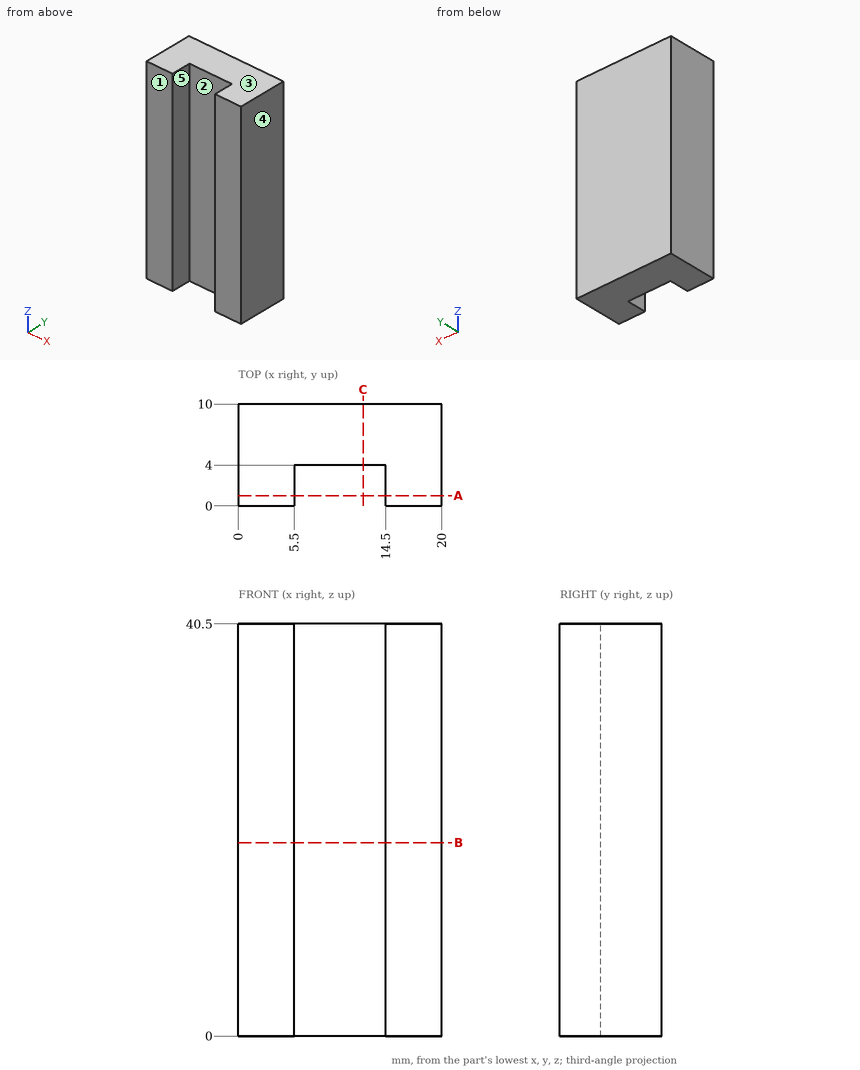
Study the drawing (mm; zero at the part's minimum x, y, z) and answer. A direction names the side the tool comes from. Coordinates: 2 decimals unless noted, no trailing zeros. Write each loop counter-clockwise with the first axis right and the second up, starting at its lowest first coordinate (ties: lowest second). Pieces come first, ordered by that corner, then holes. Notation, with made-up numbers: (49.25, -16.5) -> (76.25, -16.5) arc R20 cw to (76.25, 5.5) -> close; hole circle Ø5 at (20.25, 40). An arc over 180 degrees is marked (long way). Write each question's results on one line, items separated by ' | '. Start each with the question number.
1) A cutting plane is placed at C-C (x = 12.25). Determine the outline of the cut face in (y, z), then the cut area to 3 significant figures.
2) For a pull along X with two mould halves and no side action, classify the marked faces 3, 4 and 5 as +X half, -X half, draft (parallel to the pull), parting line (faces both ways), or undercut.
3) Straight lines are drawn through the part: probe 1 along X at (y, z) = (3.5, 27); probe 2 along Y at (x, z) = (6.5, 19). For each, find the intervals that lie inside material, in ascending order.
4) A cutting plane is placed at A-A (y = 1). Determine the outline of the cut face in (x, z).
5) A cutting plane is placed at B-B (z = 19). Determine the outline of the cut face in (x, y), then the cut area to 3 significant figures.
6) Flat-ended cylindrical pins translate along their axes: pin 1 Ø3 at (x, y) = (13.5, 6) entering from -Z; pin 2 Ø4.5 at (x, z) = (8, 22.5) entering from -Y. Find the tip coordinate at first contact, or state that the pin passes through.
7) A tool of negligible diameter and unlimited length cuts with its end or side. For the marked faces 1 and 2, from which of +Z, -Z, +X, -X, +Y, -Y can it reach the whole face along a straight path? Write none if from no direction.
Values follow:
1) outline: (4, 0) -> (10, 0) -> (10, 40.5) -> (4, 40.5) -> close | area: 243 mm²
2) face 3: draft | face 4: +X half | face 5: undercut
3) probe 1: 0 to 5.5, 14.5 to 20 | probe 2: 4 to 10
4) outline: (0, 0) -> (5.5, 0) -> (5.5, 40.5) -> (0, 40.5) -> close; (14.5, 0) -> (20, 0) -> (20, 40.5) -> (14.5, 40.5) -> close
5) outline: (0, 0) -> (5.5, 0) -> (5.5, 4) -> (14.5, 4) -> (14.5, 0) -> (20, 0) -> (20, 10) -> (0, 10) -> close | area: 164 mm²
6) pin 1: z = 0 | pin 2: y = 4
7) face 1: +Z, -Z, +X, -X, -Y | face 2: +Z, -Z, -Y
